from build123d import *

# Parameters (mm, degrees)
SKETCH_2_W          = 169
SKETCH_2_H          = 100
EXTRUDE_2_DEPTH     = 122
SKETCH_6_W          = 165
SKETCH_6_H          = 118
CUT_EXTRUDE_3_DEPTH = 98
SKETCH_7_W          = 40
SKETCH_7_H          = 40
CUT_EXTRUDE_4_DEPTH = 215.347848135
SKETCH_8_R          = 3
CUT_EXTRUDE_5_DEPTH = 10
SKETCH_9_R          = 3
CUT_EXTRUDE_6_DEPTH = 10
SKETCH_10_R         = 3
CUT_EXTRUDE_7_DEPTH = 10


with BuildPart() as part:
    # ｽｹｯﾁ2 → ﾎﾞｽ - 押し出し2 (new body)
    with BuildSketch(Plane(origin=(0, 0, 0), x_dir=(1, 0, 0), z_dir=(0, 1, 0))):
        Rectangle(SKETCH_2_W, SKETCH_2_H)
    extrude(amount=EXTRUDE_2_DEPTH)

    # ｽｹｯﾁ6 → ｶｯﾄ - 押し出し3 (cut)
    with BuildSketch(Plane.XY.offset(50)):
        with Locations((0, 61)):
            Rectangle(SKETCH_6_W, SKETCH_6_H)
    extrude(amount=-CUT_EXTRUDE_3_DEPTH, mode=Mode.SUBTRACT)

    # ｽｹｯﾁ7 → ｶｯﾄ - 押し出し4 (cut, through all)
    with BuildSketch(Plane(origin=(84.5, 0, 0), x_dir=(0, 0, -1), z_dir=(1, 0, 0))):
        with Locations((30, 102)):
            Rectangle(SKETCH_7_W, SKETCH_7_H)
    extrude(amount=-CUT_EXTRUDE_4_DEPTH, mode=Mode.SUBTRACT)

    # ｽｹｯﾁ8 → ｶｯﾄ - 押し出し5 (cut)
    with BuildSketch(Plane(origin=(0, 2, 0), x_dir=(1, 0, 0), z_dir=(0, 1, 0))):
        with Locations(Location((-72, -35, 0), (0, 0, 270))):
            Circle(SKETCH_8_R)
        with Locations(Location((72, -35, 0), (0, 0, 270))):
            Circle(SKETCH_8_R)
    extrude(amount=-CUT_EXTRUDE_5_DEPTH, mode=Mode.SUBTRACT)

    # ｽｹｯﾁ9 → ｶｯﾄ - 押し出し6 (cut)
    with BuildSketch(Plane.XY.offset(-48)):
        with Locations((-72, 67)):
            Circle(SKETCH_9_R)
        with Locations((72, 69)):
            Circle(SKETCH_9_R)
    extrude(amount=-CUT_EXTRUDE_6_DEPTH, mode=Mode.SUBTRACT)

    # ｽｹｯﾁ10 → ｶｯﾄ - 押し出し7 (cut)
    with BuildSketch(Plane(origin=(84.5, 0, 0), x_dir=(0, 0, -1), z_dir=(1, 0, 0))):
        with Locations((-2.5, 69)):
            Circle(SKETCH_10_R)
    extrude(amount=-CUT_EXTRUDE_7_DEPTH, mode=Mode.SUBTRACT)


solid = part.part
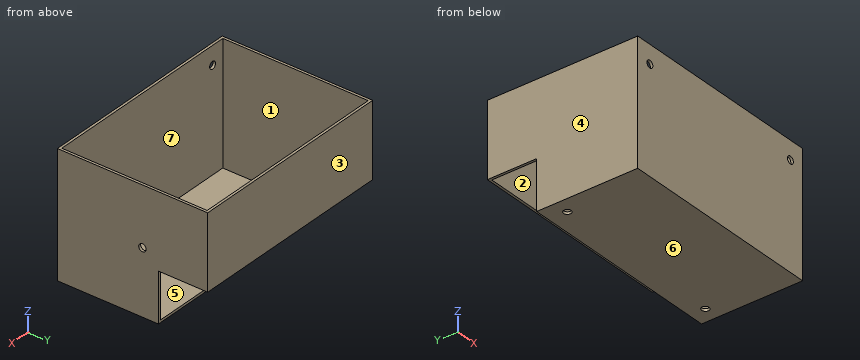
For this review, take the finished solid that the model builds, in its own axes (mm). Face numbers are marked on the shaded views. A direction names the side the tool comes from. Round coordinates to 2 decimals unless told otherwise and drop trailing zeros. Write each loop counter-clockwise with the first axis right and the second up, starting at its lowest first coordinate (ties: lowest second). Pieces come first, ordered by that corner, then holes. Notation, with made-up numbers: (59.25, 74) -> (98.25, 74) arc R6 cw to (98.25, 79) -> close; hole circle Ø4 at (-21.75, 16). An arc over 180 degrees is marked (long way). Put each result on its own line as item: value.
Q1. To check wall thickness, follow L1, parallel to Y at x = 72, z = -49.15; L2, parallel to Y at x = 51, z = 38; L3, parallel to X at y = 113.5, z = -7.5. State the ranges of each line that lie inside material, in increasing order. Write a range as [from, to].
Determined:
L1: y = [0, 66], [72, 82]
L2: y = [0, 2], [120, 122]
L3: x = [-84.5, -82.5], [82.5, 84.5]
Q2. Consider section A-A on x = -14. State the section outline as (y, z) points, and give its area (3 significant figures).
Determined:
outline: (0, -50) -> (82, -50) -> (82, -48) -> (2, -48) -> (2, 50) -> (0, 50) -> close; (120, -10) -> (122, -10) -> (122, 50) -> (120, 50) -> close
area: 480 mm^2
Q3. Consider section C-C on x = 72. State the section outline as (y, z) points, and give its area (3 significant figures).
Determined:
outline: (0, -50) -> (66, -50) -> (66, -48) -> (2, -48) -> (2, 32) -> (0, 32) -> close; (0, 38) -> (2, 38) -> (2, 50) -> (0, 50) -> close; (72, -50) -> (82, -50) -> (82, -48) -> (72, -48) -> close; (120, -10) -> (122, -10) -> (122, 50) -> (120, 50) -> close
area: 456 mm^2
Q4. Consider section D-D on y = 76.5. State the section outline as (x, z) points.
Determined:
outline: (-84.5, -50) -> (84.5, -50) -> (84.5, 50) -> (82.5, 50) -> (82.5, -48) -> (-82.5, -48) -> (-82.5, 50) -> (-84.5, 50) -> close
Q5. Clearance check with flat-ended pins moving along their axes: pin 1 Ø3.5 at (x, y) = (72, 69) entering from +Z; pin 2 Ø4 at (x, z) = (43, -30) entering from +Y. State where each tip first meets the part, or that it passes through.
Determined:
pin 1: passes through
pin 2: stops at y = 2
Q6. Machinability: for the marked faces 5, 6 and 7, which of the approach directions +Z, -Z, +X, -X, +Y, -Y give a long, thin tool a straight path to every point of the face, cutting with its end or side? Answer none if there is none.
Determined:
face 5: +Z, +Y
face 6: -Z, +X, -X, +Y, -Y
face 7: +Z
Q7. The part is to be moulded in two halves that separate along Y. For the marked faces 1, 2, 3 and 4, say which applies: released by +Y, released by -Y, zero draft, split by the parting line, or undercut.
Determined:
face 1: undercut
face 2: undercut
face 3: released by +Y
face 4: zero draft
Q8. Consider section B-B on z = 35. State the section outline as (x, y) points, and give its area (3 significant figures).
Determined:
outline: (-84.5, 0) -> (-75, 0) -> (-75, 2) -> (-82.5, 2) -> (-82.5, 120) -> (82.5, 120) -> (82.5, 2) -> (75, 2) -> (75, 0) -> (84.5, 0) -> (84.5, 122) -> (-84.5, 122) -> close; (-69, 0) -> (69, 0) -> (69, 2) -> (-69, 2) -> close
area: 1,120 mm^2
